Can you work these out from the drawing? Everything is in mm from the part's minimum corner. A direction names the side the tool comes from. Round coordinates to 2 decimals unless told otherwise and drop trailing zeros. Loops run counter-clockwise (first coordinate to the right, second up) from the corner with the lowest first, then second, coordinate; pieces in that order, holes last. Notation, with made-up numbers: M 18.25,54.25 L 75.25,54.25 A33 cw 75.25,84.25 Z; hole C 54,46 d3. An arc over 180 degrees is marked long. Return JSON: item names as keys, results as strings. Group by question number.
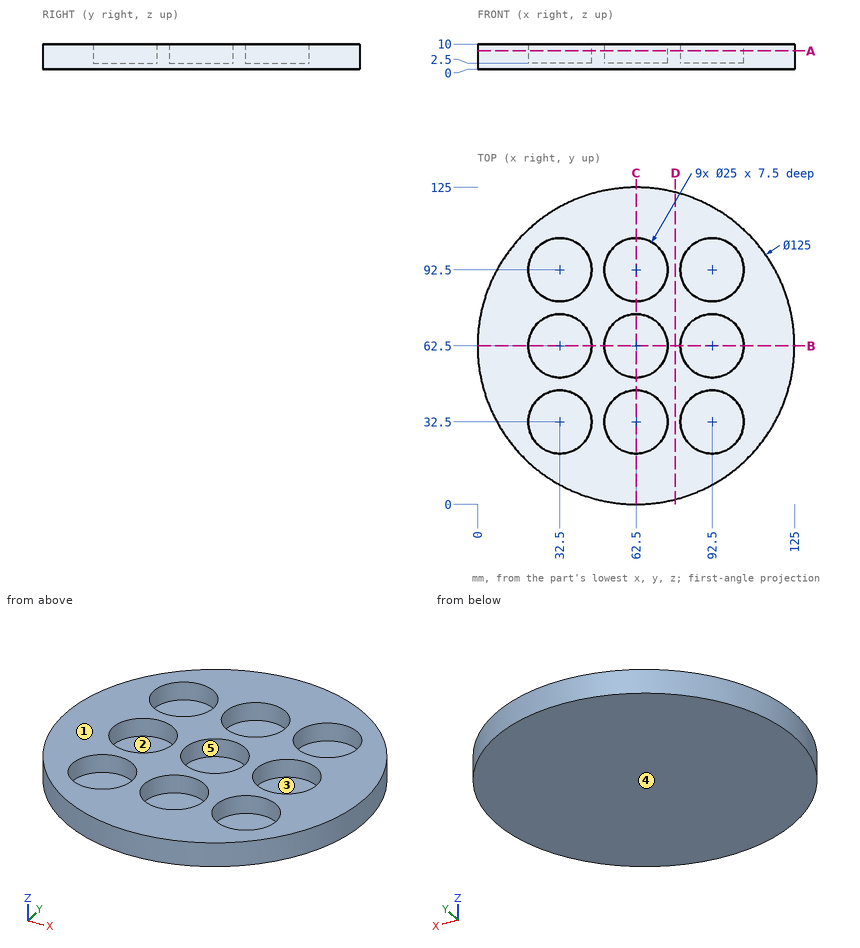
1. I'm going to push flat-ended pins straight in: pin 1 Ø20 at (x, y) = (32.5, 62.5) entering from +Z; pin 2 Ø20 at (x, y) = (35.5, 31.5) entering from +Z; pin 3 Ø2 at (y, z) = (16, 5.5) entering from +X; pin 4 Ø2 at (x, z) = (104, 4) entering from -Y. Where does each tip first touch, or does it pass through?
2. If we section it at B-B, the plane y = 62.5: Please give me the cut outline in (x, z).
3. We'd pull the mould along X, two halves only. Please class the marked faces 1, 2 and 3: +X half, -X half, draft (parallel to the pull), parting line (faces both ways), or undercut.
4. I need wall thicknesses on probe 1 along Y at (x, z) = (62.5, 8); probe 2 along Y at (x, z) = (95, 4.75); probe 3 along X at (y, z) = (92.5, 8). Which ranges of each line are inside material? Lowest first, please.
5. On a 3-axis mill with a long thin cutter (end or side, diameter ignored), from which of +Z, -Z, +X, -X, +Y, -Y can I reach the whole of each face in a straight line? I mean the marked faces 4 and 5. Say none if no direction works.
6. If we section it at D-D, the plane x = 78: Please give me the cut outline in (y, z), then the cut area to 3 significant figures.
7. If we section it at A-A, the plane z = 7.25: Give the number of separate pieces and of enclosed holes in the cut face, then the cut area to 3 significant figures.
Geometry results:
{
 "1": {"pin 1": "z = 2.5", "pin 2": "z = 10", "pin 3": "x = 105.35", "pin 4": "y = 14.9"},
 "2": {"outline": "M 0,0 L 125,0 L 125,10 L 105,10 L 105,2.5 L 80,2.5 L 80,10 L 75,10 L 75,2.5 L 50,2.5 L 50,10 L 45,10 L 45,2.5 L 20,2.5 L 20,10 L 0,10 Z"},
 "3": {"face 1": "draft", "face 2": "undercut", "face 3": "undercut"},
 "4": {"probe 1": "0 to 20, 45 to 50, 75 to 80, 105 to 125", "probe 2": "9.11 to 20.25, 44.75 to 50.25, 74.75 to 80.25, 104.75 to 115.89", "probe 3": "7.67 to 20, 45 to 50, 75 to 80, 105 to 117.33"},
 "5": {"face 4": "-Z, +X, -X, +Y, -Y", "face 5": "+Z"},
 "6": {"outline": "M 1.95,0 L 123.05,0 L 123.05,10 L 1.95,10 Z", "area": "1,210 mm^2"},
 "7": {"separate pieces": "1", "enclosed holes": "9", "area": "7,850 mm^2"}
}
